from build123d import *

# Parameters (mm, degrees)
F1_DEPTH = 25
F2_R     = 1


# Not quite as in the source:
# - a feature names something its author has since deleted; it is built from what else it names


with BuildPart() as f1:
    # F0 (on Top) → F1 (new body)
    with BuildSketch(Plane.XY):
        Polygon((0, -2), (0, 0), (-36.5, 0), (-36.5, 10.3007538181), (-38.5, 8.4454781792), (-38.5, -2), (-15.248538491, -2), (-12, -2), align=None)
        Polygon((36.5, 0), (0, 0), (0, -2), (12, -2), (15.248538491, -2), (38.5, -2), (38.5, 8.4454781792), (36.5, 10.3007538181), align=None)
        Polygon((-38.5, 8.4454781792), (-36.5, 10.3007538181), (-36.5, 13.0287654926), (-38.5, 11.1734898537), align=None)
        Polygon((-30.5484807652, -16.4916614154), (-12, -2), (-15.248538491, -2), (-30.3854576709, -13.8262573849), (-45.844322202, 1.6326071462), (-47.3116243561, 0.2714821755), align=None)
        Polygon((15.248538491, -2), (12, -2), (30.5484807652, -16.4916614154), (47.3116243561, 0.2714821755), (45.844322202, 1.6326071462), (30.3854576709, -13.8262573849), align=None)
        Polygon((36.5, 13.0287654926), (36.5, 10.3007538181), (38.5, 8.4454781792), (38.5, 11.1734898537), align=None)
        Polygon((-45.844322202, 1.6326071462), (-38.5, 8.4454781792), (-38.5, 11.1734898537), (-47.259531868, 3.0478168121), align=None)
        Polygon((38.5, 11.1734898537), (38.5, 8.4454781792), (45.844322202, 1.6326071462), (47.259531868, 3.0478168121), align=None)
        Polygon((-47.3116243561, 0.2714821755), (-45.844322202, 1.6326071462), (-47.259531868, 3.0478168121), (-48.726834022, 1.6866918414), align=None)
        Polygon((45.844322202, 1.6326071462), (47.3116243561, 0.2714821755), (48.726834022, 1.6866918414), (47.259531868, 3.0478168121), align=None)
    extrude(amount=F1_DEPTH)

    # F2
    f2_edges = [f1.edges().sort_by_distance(p)[0] for p in [
        (-36.5, 0, 12.5),
        (-38.5, -2, 12.5),
        (-15.248538, -2, 12.5),
        (15.248538, -2, 12.5),
        (30.385458, -13.826257, 12.5),
        (38.5, -2, 12.5),
        (38.5, 8.445478, 12.5),
        (45.844322, 1.632607, 12.5),
        (12, -2, 12.5),
        (30.548481, -16.491661, 12.5),
        (36.5, 13.028765, 12.5),
        (36.5, 0, 12.5),
        (48.726834, 1.686692, 12.5),
        (-45.844322, 1.632607, 12.5),
        (-48.726834, 1.686692, 12.5),
        (-36.5, 13.028765, 12.5),
        (-30.548481, -16.491661, 12.5),
        (-12, -2, 12.5),
        (-30.385458, -13.826257, 12.5),
        (-38.5, 8.445478, 12.5),
    ]]
    fillet(f2_edges, radius=F2_R)


solid = f1.part
Geometry check sheet. Reference: the model listing, model coordinates, mm. A direction names the side the tool comes from. Give positions to 0.01 mm unless a question says otherwise; leave off trailing zeros. Order: outer loops, then holes, each group sorted by start corner. A loop starts at its lowest first (then second) coordinate and runs counter-clockwise, first axis right, second up.
1. Draft check along Y on faces 1 (the face through (-17.2, -2.7, 12.7)), 2 (the face through (37.11, 11.66, 12.68)), 3 (the face through (-37.96, -6.25, 12.32)), 4 (the face through (39.47, -7.57, 12.32)). Enter one of: pulls with the +Y half, pulls with the -Y half, needs draft (parallel to the pull), parting line crosses it, or undercut.
Completed:
face 1: undercut
face 2: pulls with the +Y half
face 3: undercut
face 4: pulls with the -Y half
2. Depth check by flat-ended pin: pin 1 (6 mm diameter, centred on x = -29.5, z = 8, fed in from +Y); pin 2 (3 mm diameter, centred on y = -8.5, z = 9.5, fed in from -X); pin 3 (3 mm diameter, centred on y = 4, z = 7.5, fed in from -X); pin 4 (2 mm diameter, centred on y = 1, z = 17, fed in from -X). Enter the tip coordinate at first touch or a pass-through.
Completed:
pin 1: stops at y = 0
pin 2: stops at x = -40.04
pin 3: stops at x = -47.85
pin 4: stops at x = -48.29
3. Sectioned sample at B-B (y = -9.25). Record the boundary of the cut face in (x, z).
Completed:
outline: (-37.79, 0) - (-34.96, 0) - (-34.96, 25) - (-37.79, 25) - close; (-24.53, 0) - (-21.28, 0) - (-21.28, 25) - (-24.53, 25) - close; (21.28, 0) - (24.53, 0) - (24.53, 25) - (21.28, 25) - close; (34.96, 0) - (37.79, 0) - (37.79, 25) - (34.96, 25) - close
4. Scan lines: line 1 (X direction, y = 0.5, z = 11.5); line 2 (X direction, y = -0.25, z = 16.75); line 3 (X direction, y = -11.5, z = 5.75). Record each from-to range of solid material in increasing order.
Completed:
line 1: x = -47.54 to -44.71, -38.5 to -36.37, 36.37 to 38.5, 44.71 to 47.54
line 2: x = -46.79 to -43.96, -38.5 to 38.5, 43.96 to 46.79
line 3: x = -35.54 to -32.71, -27.41 to -24.16, 24.16 to 27.41, 32.71 to 35.54
5. Sectioned sample at A-A (x = -28). Record the boundary of the cut face in (y, z).
Completed:
outline: (-14.5, 0) - (-11.96, 0) - (-11.96, 25) - (-14.5, 25) - close; (-2, 0) - (0, 0) - (0, 25) - (-2, 25) - close
6. Sectioned sample at D-D (x = 33.5). Record the boundary of the cut face in (y, z).
Completed:
outline: (-13.54, 0) - (-10.71, 0) - (-10.71, 25) - (-13.54, 25) - close; (-2, 0) - (0, 0) - (0, 25) - (-2, 25) - close
7. Sectioned sample at C-C (z = 11.75). State how many separate pieces and enclosed holes the cut face has, then the cut area to 3 significant figures.
Completed:
separate pieces: 1
enclosed holes: 2
area: 434 mm2
8. Access from +Z, -Z, +X, -X, +Y, -Y to the whole of each face (thin tool, end or side, straight path). Record for faces 5 (the face through (-36.5, 6, 12)), 6 (the face through (0, -1, 0)), 7 (the face through (0, -1, 25)), 8 (the face through (-42.666, 4.581, 12.325)), 9 (the face through (0, -2, 12)).
Completed:
face 5: +Z, -Z, +Y
face 6: -Z, +X, -X, +Y, -Y
face 7: +Z, +X, -X, +Y, -Y
face 8: +Z, -Z
face 9: +Z, -Z, -Y
